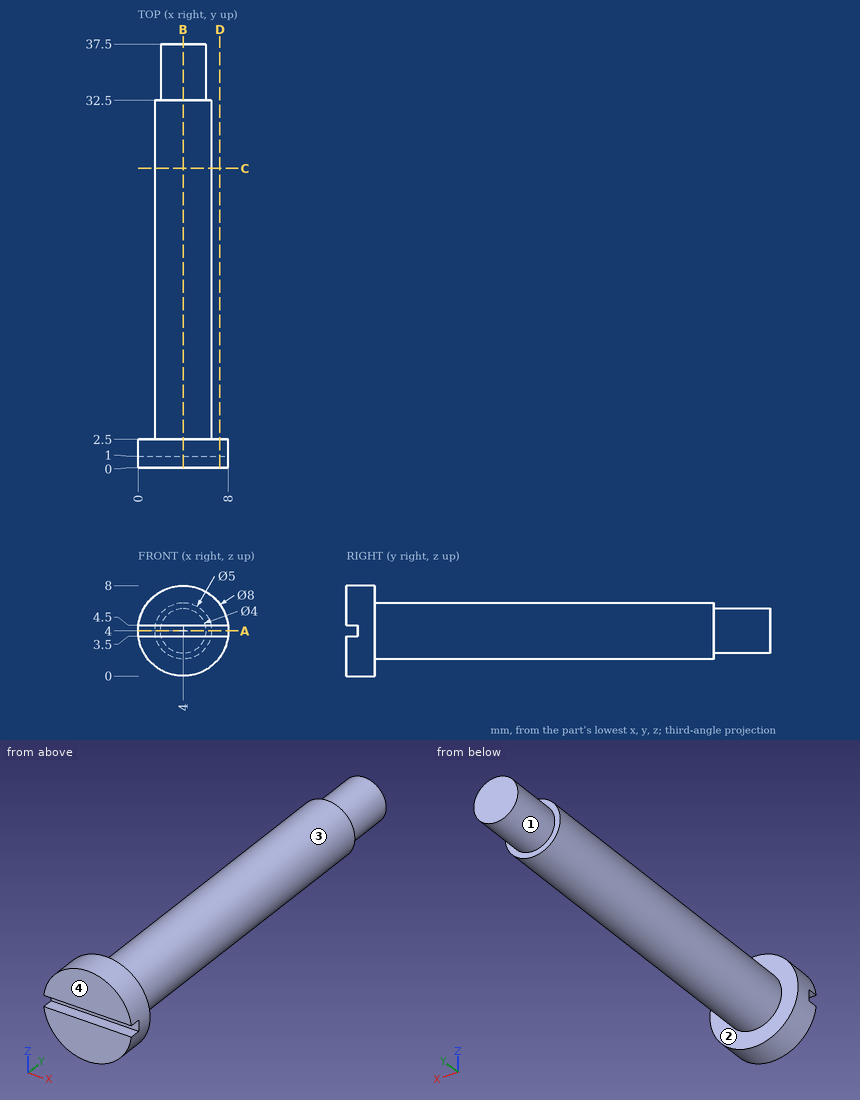
Check sheet for the drawn part. Datum: minimum x, y, z corner. Units: mm. A direction names the side the tool comes from. Coordinates: 2 decimals unless noted, no trailing zeros. Loops run counter-clockwise (first coordinate to the right, second up) from the corner with the lowest first, then second, coordinate; pieces in that order, holes last. Notation, with made-up numbers: (-39, 10) -> (13, 10) arc R21 ccw to (13, 39) -> close; hole circle Ø5 at (88.25, -25.5). An arc over 180 degrees is marked (long way). Write each question's results on one line, items separated by ' | '.
Item 1: Mould release check, pull along Z, two halves, no side actions. Record for the marked faces 1 and 2: +Z half, -Z half, draft (parallel to the pull), parting line (faces both ways), or undercut.
Found:
face 1: parting line | face 2: draft
Item 2: Section check B-B, the plane x = 4. Enter the section's corners in (y, z), plus the area to 3 significant figures.
Found:
outline: (0, 0) -> (2.5, 0) -> (2.5, 1.5) -> (32.5, 1.5) -> (32.5, 2) -> (37.5, 2) -> (37.5, 6) -> (32.5, 6) -> (32.5, 6.5) -> (2.5, 6.5) -> (2.5, 8) -> (0, 8) -> (0, 4.5) -> (1, 4.5) -> (1, 3.5) -> (0, 3.5) -> close | area: 189 mm2
Item 3: Material ranges on L1, parallel to Y at x = 7, z = 6.5; L2, parallel to Y at x = 5, z = 2; L3, parallel to X at y = 5.5, z = 5.5, recorded low to high.
Found:
L1: y = 0 to 2.5 | L2: y = 0 to 32.5 | L3: x = 2 to 6
Item 4: Gauge pin test, flat ends, axial feed: pin 1 (2 mm diameter, centred on x = 6, y = 29.5, fed in from -Z); pin 2 (1.1 mm diameter, centred on x = 2, z = 4, fed in from -Y); pin 3 (3 mm diameter, centred on y = 11, z = 3.5, fed in from -X); pin 4 (2 mm diameter, centred on y = 9, z = 6, fed in from -X). Record the tip position at first contact, or that the pin passes through.
Found:
pin 1: stops at z = 1.71 | pin 2: stops at y = 0 | pin 3: stops at x = 1.5 | pin 4: stops at x = 1.71
Item 5: Section check D-D, the plane x = 7.25. Enter the section's corners in (y, z).
Found:
outline: (0, 1.67) -> (2.5, 1.67) -> (2.5, 6.33) -> (0, 6.33) -> (0, 4.5) -> (1, 4.5) -> (1, 3.5) -> (0, 3.5) -> close
Item 6: Section check A-A, the plane z = 4. Enter the section's corners in (x, y), plus the area to 3 significant figures.
Found:
outline: (0, 1) -> (8, 1) -> (8, 2.5) -> (6.5, 2.5) -> (6.5, 32.5) -> (6, 32.5) -> (6, 37.5) -> (2, 37.5) -> (2, 32.5) -> (1.5, 32.5) -> (1.5, 2.5) -> (0, 2.5) -> close | area: 182 mm2
Item 7: Section check C-C, the plane y = 26.5. Enter the section's corners in (x, z), plus the area to 3 significant figures.
Found:
outline: circle Ø5 at (4, 4) | area: 19.6 mm2
Item 8: Tool access check on the marked faces 3 and 4. Record the directions out of +Z, -Z, +X, -X, +Y, -Y that give a thin tool (end or side, any length) a straight path to the whole face; none if there is none.
Found:
face 3: +Y | face 4: +Z, -Z, +X, -X, -Y
